from build123d import *

# Parameters (mm, degrees)
SKETCH2_W                           = 28
SKETCH2_H                           = 18
SKETCH2_W_2                         = 23.6
SKETCH2_H_2                         = 12.8
SERVO_MOUNT_CRADLE_DEPTH            = 4
SKETCH3_W                           = 40
SKETCH3_H                           = 10
REAR_WALL_CLEARANCE_U_BRACKET_DEPTH = 18.117242769


with BuildPart() as part:
    # Sketch2 → Servo_mount_cradle (new body)
    with BuildSketch(Plane.XY):
        Rectangle(SKETCH2_W, SKETCH2_H)
        Rectangle(SKETCH2_W_2, SKETCH2_H_2, mode=Mode.SUBTRACT)
    extrude(amount=SERVO_MOUNT_CRADLE_DEPTH)

    # Sketch3 → Rear_wall_clearance_U_bracket (cut, through all)
    with BuildSketch(Plane.XY):
        with Locations((0, 11.4)):
            Rectangle(SKETCH3_W, SKETCH3_H)
    extrude(amount=REAR_WALL_CLEARANCE_U_BRACKET_DEPTH, mode=Mode.SUBTRACT)


solid = part.part
Design review of the part built by this model. Coordinates are the model's own, in mm. A direction names the side the tool comes from. Coordinates: 2 decimals unless noted, no trailing zeros. Loops run counter-clockwise (first coordinate to the right, second up) from the corner with the lowest first, then second, coordinate; pieces in that order, holes last. Notation, with made-up numbers: (16.5, 24) -> (29.5, 24) arc R17 cw to (29.5, 41) -> close; hole circle Ø1 at (64, 75). An arc over 180 degrees is marked (long way). Use a Markdown table: item, result. Add a question column.
Item 1: Clearance check with flat-ended pins moving along their axes: P1, Ø4, axis at x = -9, y = 3.5, coming from the -Z side; P2, Ø1, axis at x = -5.5, z = 0.5, coming from the +Y side. State where each tip first meets the part, or that it passes through.
Item 2: We need section C-C, the plane x = -8.75. Write out the cut boundary in (y, z), and give its area (3 significant figures).
Item 3: We need section A-A, the plane y = -5.75. Write out the cut boundary in (x, z), and give its area (3 significant figures).
Item 4: Machinability: for faces 1 (the flat face through (13, 6.4, 2)), 2 (the flat face through (-11.8, 0, 2)), which of the approach directions +Z, -Z, +X, -X, +Y, -Y give a long, thin tool a straight path to every point of the face, cutting with its end or side? Answer none if there is none.
Item 5: Wall thickness on L1, parallel to X at y = 3.25, z = 2.8; L2, parallel to Y at x = -7, z = 2.35: over which ranges is each line inside the solid? List them lowest first. Write a range as from..to.
Item 6: We need section B-B, the plane z = 3.5. Write out the cut boundary in (x, y).
Numbers:
| question | item | result |
|---|---|---|
| 1 | P1 | passes through |
| 1 | P2 | stops at y = -6.4 |
| 2 | outline | (-9, 0) -> (-6.4, 0) -> (-6.4, 4) -> (-9, 4) -> close |
| 2 | area | 10.4 mm^2 |
| 3 | outline | (-14, 0) -> (-11.8, 0) -> (-11.8, 4) -> (-14, 4) -> close; (11.8, 0) -> (14, 0) -> (14, 4) -> (11.8, 4) -> close |
| 3 | area | 17.6 mm^2 |
| 4 | face 1 | +Z, -Z, +X, -X, +Y |
| 4 | face 2 | +Z, -Z, +Y |
| 5 | L1 | x = -14..-11.8, 11.8..14 |
| 5 | L2 | y = -9..-6.4 |
| 6 | outline | (-14, -9) -> (14, -9) -> (14, 6.4) -> (11.8, 6.4) -> (11.8, -6.4) -> (-11.8, -6.4) -> (-11.8, 6.4) -> (-14, 6.4) -> close |
